from build123d import *

# Parameters (mm, degrees)
SKETCH_1_W             = 38
SKETCH_1_H             = 40
SKETCH_1_R             = 9
SM_BASE_FLANGE_1_DEPTH = 2
SM_EDGE_FLANGE_1_DEPTH = 38
FILLET_1_R             = 10


# Sheet-metal steps are written as plain solids
with BuildPart() as part:
    # Sketch 1 → 基体-法兰1 (new body)
    with BuildSketch(Plane.XY):
        with Locations((0, -5)):
            Rectangle(SKETCH_1_W, SKETCH_1_H)
        Circle(SKETCH_1_R, mode=Mode.SUBTRACT)
    extrude(amount=-SM_BASE_FLANGE_1_DEPTH)

    # 边线-法兰1 section (across the edge) → 边线-法兰1 (add)
    with BuildSketch(Plane(origin=(19, -28, -2), x_dir=(0, 1, 0), z_dir=(-1, 0, 0))):
        with BuildLine():
            Line((-2, 3), (-2, 18))
            Line((-2, 18), (0, 18))
            Line((0, 18), (0, 3))
            ThreePointArc((0, 3), (0.878679656, 0.878679656), (3, 0))
            Line((3, 0), (3, -2))
            ThreePointArc((3, -2), (-0.535533906, -0.535533906), (-2, 3))
        make_face()
    extrude(amount=SM_EDGE_FLANGE_1_DEPTH)

    # 圆角1
    fillet_1_edges = [part.edges().sort_by_distance(p)[0] for p in [
        (19, -29, -20),
        (-19, -29, -20),
        (19, 15, -1),
        (-19, 15, -1),
    ]]
    fillet(fillet_1_edges, radius=FILLET_1_R)


solid = part.part
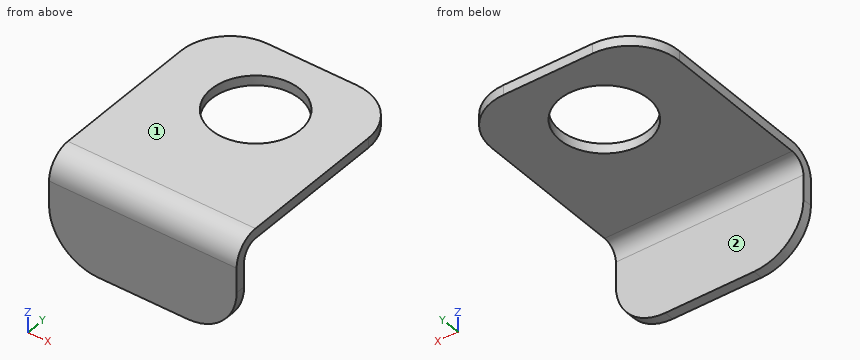
Geometry check sheet. Reference: the model listing, model coordinates, mm. Face numbers are marked on the shaded views. A direction names the side the tool comes from. Round coordinates to 2 decimals unless told otherwise and drop trailing zeros. Order: outer loops, then holes, each group sorted by start corner. A loop starts at its lowest first (then second) coordinate and runs counter-clockwise, first axis right, second up. Notation, with made-up numbers: M 6.5,-19.5 L 25.5,-19.5 A26 cw 25.5,3.5 Z; hole C 87,50 d10. An arc over 180 degrees is marked long. Write each question's results on one line, items separated by ' | '. Start each with the question number.
1. Cross-section at D-D on x = 14.5. Record the boundary of the cut face in (y, z).
2. Cross-section at A-A on y = 0. Record the boundary of the cut face in (x, z), plus the area to 3 significant figures.
3. Material ranges on L1, parallel to Z at x = -14, y = -4.5; L2, parallel to Y at x = -2, z = -16; L3, parallel to Y at x = 0, z = -0.85, recorded low to high. Write a range as from..to.
4. Set-up check for the marked faces 1 and 2: record each of +Z, -Z, +X, -X, +Y, -Y from which the full face is reachable in a straight line by a thin tool's end or side.
5. Go/stop test with flat-tipped pins: P1, Ø12, axis at y = -16.5, z = -12.5, coming from the -X side; P2, Ø3, axis at x = 4, y = -21, coming from the -Z side; P3, Ø3, axis at x = -7, y = 9, coming from the +Z side; P4, Ø6, axis at x = 13, z = -2.5, coming from the +Y side. Record where each tip stops, or that it passes through.
6. Cross-section at B-B on x = 0. Record the boundary of the cut face in (y, z), plus the area to 3 significant figures.
7. Cross-section at C-C on y = -14.5. Record the boundary of the cut face in (x, z).
Resolved:
1) outline: M -30,-18.35 L -28,-18.35 L -28,-5 A3 cw -25,-2 L 13.35,-2 L 13.35,0 L -25,0 A5 ccw -30,-5 Z
2) outline: M -19,-2 L -9,-2 L -9,0 L -19,0 Z; M 9,-2 L 19,-2 L 19,0 L 9,0 Z | area: 40.0 mm2
3) L1: -2..0 | L2: -30..-28 | L3: -27.79..-9, 9..15
4) face 1: +Z, +X, -X, +Y, -Y | face 2: -Z, +X, -X, +Y
5) P1: through | P2: z = -2 | P3: z = 0 | P4: y = 14.95
6) outline: M -30,-20 L -28,-20 L -28,-5 A3 cw -25,-2 L -9,-2 L -9,0 L -25,0 A5 ccw -30,-5 Z; M 9,-2 L 15,-2 L 15,0 L 9,0 Z | area: 86.6 mm2
7) outline: M -19,-2 L 19,-2 L 19,0 L -19,0 Z
